Geometry: final body of the model. Coordinates: model frame, mm. Face numbers are marked on the shaded views. Give positions to 0.01 mm unless a question says otherwise; leave off trailing zeros. Write each loop counter-clockwise with the first axis right and the second up, starting at its lowest first coordinate (ties: lowest second). Pieces come first, ordered by that corner, then holes. Notation, with made-up numbers: M 42,3.5 L 55,3.5 A29 ccw 55,35.5 Z; hole C 52.5,44 d11. An arc over 180 degrees is marked long. Use a Markdown table: item, result. Add a question column.
(1) Cut plane D-D (x = -16). Output: boundary loops of the cut face in (y, z).
(2) Pin query (flat end, axial travel): pin 1 Ø3 at (x, z) = (-16.5, -17) entering from -Y; pin 2 Ø2.5 at (x, z) = (7.5, -10) entering from -Y; pin 3 Ø5 at (x, z) = (-7.5, -10) entering from +Y; pin 4 Ø2 at (x, z) = (-3.5, -17) entering from -Y. Return the tip coordinate at first contact, or that it passes through.
(3) Material intervals for L1, parallel to X at y = 1.25, z = 10; L2, parallel to Z at x = -3.5, y = 2.05; L3, parallel to X at y = 0.8, z = -16, sorted ascending.
(4) Cut plane B-B (z = -10). Output: boundary loops of the cut face in (x, y), plus the area to 3 significant figures.
(5) Draft query along Z for the marked faces 1, 2 and 3. Return one class per face: released by +Z, released by -Z, zero draft, split by the parting line, or undercut.
(6) Cut plane C-C (y = 1.7). State how many separate pieces and enclosed holes the cut face has, plus the area to 3 significant figures.
(7) Cut plane A-A (x = 7.5). Output: boundary loops of the cut face in (y, z).
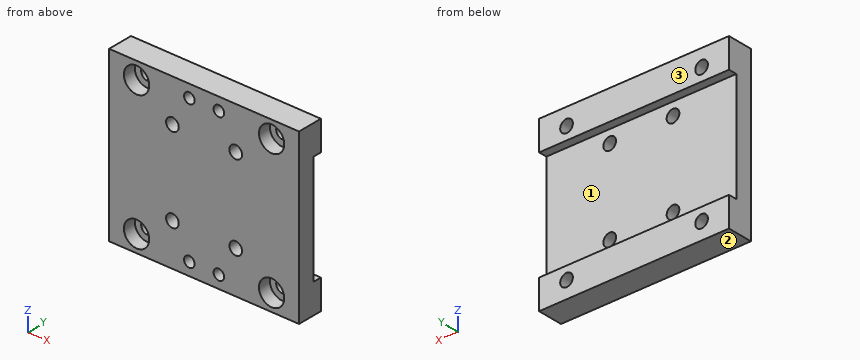
```python
from build123d import *

# Parameters (mm, degrees)
SKETCH_2_W                = 45
SKETCH_2_H                = 33
SKETCH_2_R                = 1.5
EXTRUDE_1_DEPTH           = 6
SKETCH_3_W                = 45
SKETCH_3_H                = 3.5
EXTRUDE_2_DEPTH           = 6
SKETCH_20_W               = 45
SKETCH_20_H               = 27.5
CUT_EXTRUDE_5_DEPTH       = 2
EXTRUDE_START             = -2
SKETCH_21_W               = 45
SKETCH_21_H               = 3.5
EXTRUDE_3_DEPTH           = 2
HOLE_WIZARD_3_0_3_1_D     = 3
HOLE_WIZARD_3_0_3_1_DEPTH = 6
HOLE_WIZARD_M3_2_D        = 2.5
HOLE_WIZARD_M3_2_DEPTH    = 4
HOLE_WIZARD_M3_2_TIP      = 0.751075774
HOLE_WIZARD_1_D           = 3
HOLE_WIZARD_1_DEPTH       = 6
HOLE_WIZARD_1_CBORE_D     = 6
HOLE_WIZARD_1_CBORE_DEPTH = 3


with BuildPart() as part:
    # 草图2 → 凸台-拉伸1 (new body)
    with BuildSketch(Plane(origin=(0, 0, 0), x_dir=(1, 0, 0), z_dir=(0, 1, 0))):
        Rectangle(SKETCH_2_W, SKETCH_2_H)
        with Locations((-7.5, 10)):
            Circle(SKETCH_2_R, mode=Mode.SUBTRACT)
        with Locations((7.5, 10)):
            Circle(SKETCH_2_R, mode=Mode.SUBTRACT)
        with Locations((-7.5, -10)):
            Circle(SKETCH_2_R, mode=Mode.SUBTRACT)
        with Locations((7.5, -10)):
            Circle(SKETCH_2_R, mode=Mode.SUBTRACT)
    extrude(amount=EXTRUDE_1_DEPTH)

    # 草图3 → 凸台-拉伸2 (add)
    with BuildSketch(Plane.XZ):
        with Locations((0, -18.25)):
            Rectangle(SKETCH_3_W, SKETCH_3_H)
        with Locations((0, 18.25)):
            Rectangle(SKETCH_3_W, SKETCH_3_H)
    extrude(amount=-EXTRUDE_2_DEPTH)

    # 草图20 → 切除-拉伸5 (cut)
    with BuildSketch(Plane(origin=(0, 6, 0), x_dir=(1, 0, 0), z_dir=(0, 1, 0))):
        Rectangle(SKETCH_20_W, SKETCH_20_H)
    extrude(amount=-CUT_EXTRUDE_5_DEPTH, mode=Mode.SUBTRACT)

    # 草图21 → 凸台-拉伸3 (add)
    with BuildSketch(Plane.XZ.offset(-4).offset(EXTRUDE_START)):
        with Locations((0, -14.75)):
            Rectangle(SKETCH_21_W, SKETCH_21_H)
        with Locations((0, 14.75)):
            Rectangle(SKETCH_21_W, SKETCH_21_H)
    extrude(amount=EXTRUDE_3_DEPTH)

    # Ø3.0 (3) 直径孔1
    with Locations(Plane(origin=(0, 6, 0), x_dir=(1, 0, 0), z_dir=(0, 1, 0))):
        with Locations((-16, 16), (16, 16), (16, -16), (-16, -16)):
            Hole(HOLE_WIZARD_3_0_3_1_D / 2, depth=HOLE_WIZARD_3_0_3_1_DEPTH)

    # M3 螺纹孔2
    with Locations(Plane(origin=(0, 0, 0), x_dir=(-1, 0, 0), z_dir=(0, -1, 0))):
        with Locations((3.5, -17), (-3.5, -17), (-3.5, 17), (3.5, 17)):
            Hole(HOLE_WIZARD_M3_2_D / 2, depth=HOLE_WIZARD_M3_2_DEPTH)
            with Locations((0, 0, -(HOLE_WIZARD_M3_2_DEPTH + HOLE_WIZARD_M3_2_TIP / 2))):  # 118° drill point
                Cone(0, HOLE_WIZARD_M3_2_D / 2, HOLE_WIZARD_M3_2_TIP, mode=Mode.SUBTRACT)

    # 打孔尺寸(%根据)内六角圆柱头螺钉的类型1
    with Locations(Plane(origin=(0, 0, 0), x_dir=(-1, 0, 0), z_dir=(0, -1, 0))):
        with Locations((-16, 16), (16, 16), (16, -16), (-16, -16)):
            CounterBoreHole(HOLE_WIZARD_1_D / 2, HOLE_WIZARD_1_CBORE_D / 2, HOLE_WIZARD_1_CBORE_DEPTH, depth=HOLE_WIZARD_1_DEPTH)


solid = part.part
```
Answer list:
| question | item | result |
|---|---|---|
| 1 | outline | M 0,-20 L 6,-20 L 6,-17.5 L 3,-17.5 L 3,-19 L 0,-19 Z; M 0,-13 L 3,-13 L 3,-14.5 L 6,-14.5 L 6,-13 L 4,-13 L 4,13 L 6,13 L 6,14.5 L 3,14.5 L 3,13 L 0,13 Z; M 0,19 L 3,19 L 3,17.5 L 6,17.5 L 6,20 L 0,20 Z |
| 2 | pin 1 | y = 3 |
| 2 | pin 2 | through |
| 2 | pin 3 | y = 4 |
| 2 | pin 4 | y = 4.15 |
| 3 | L1 | -22.5 to -9, -6 to 6, 9 to 22.5 |
| 3 | L2 | -20 to -18.25, -15.75 to 15.75, 18.25 to 20 |
| 3 | L3 | -22.5 to -19, -13 to -4.25, -2.75 to 2.75, 4.25 to 13, 19 to 22.5 |
| 4 | outline | M -22.5,0 L -9,0 L -9,4 L -22.5,4 Z; M -6,0 L 6,0 L 6,4 L -6,4 Z; M 9,0 L 22.5,0 L 22.5,4 L 9,4 Z |
| 4 | area | 156 mm² |
| 5 | face 1 | undercut |
| 5 | face 2 | released by -Z |
| 5 | face 3 | zero draft |
| 6 | separate pieces | 1 |
| 6 | enclosed holes | 12 |
| 6 | area | 1,640 mm² |
| 7 | outline | M 0,-20 L 6,-20 L 6,-13 L 4,-13 L 4,-11.5 L 0,-11.5 Z; M 0,-8.5 L 4,-8.5 L 4,8.5 L 0,8.5 Z; M 0,11.5 L 4,11.5 L 4,13 L 6,13 L 6,20 L 0,20 Z |
